Input: part model. Units: mm. Frame: model coordinates. Face numbers are marked on the shaded views. Give positions to 0.01 mm unless a question says otherwise; leave off trailing zeros. Write each loop counter-clockwise with the first axis right and the second up, starting at its lowest first coordinate (ties: lowest second). Pieces come first, ordered by that corner, then holes. Notation, with made-up numbers: (9.5, 75) - (22.5, 75) arc R36 ccw to (22.5, 109) - close; hole circle Ø4 at (14.25, -22). An arc over 180 degrees is marked (long way). Answer as CSV lines item,"result". Start each with the question number.
Autodesk Inventor part; units mm, degrees
ref_plane "YZ Plane" through (0, 0, 0) normal (1, 0, 0) x (0, 1, 0)
ref_plane "XZ Plane" through (0, 0, 0) normal (0, 1, 0) x (-1, 0, 0)
ref_plane "XY Plane" through (0, 0, 0) normal (0, 0, 1) x (1, 0, 0)
sketch "Sketch1" plane through (0, 0, 0) normal (0, 1, 0) x (-1, 0, 0)
  arc A0 (6.35, 25.4) -> (-6.35, 25.4) centre (0, 25.4) ccw
  arc A1 (-11.43, 15.24) -> (11.43, 15.24) centre (0, 0) ccw
  arc A2 (-11.43, 15.24) -> (-6.35, 25.4) centre (-19.05, 25.4) ccw
  arc A3 (6.35, 25.4) -> (11.43, 15.24) centre (19.05, 25.4) ccw
  dimension "d0" = 25.4
  dimension "d1" = 38.1
  dimension "d2" = 12.7
extrude "Extrusion1" add sketch "Sketch1" along normal blind 3.81
sketch "Sketch2" plane through (0, 3.81, 0) normal (0, 1, 0) x (1, 0, 0)
  arc A0 (-6.35, -25.4) -> (6.35, -25.4) centre (0, -25.4) ccw
  circle A1 centre (0, -25.4) radius 1.524
  dimension "d5" = 3.048
extrude "Extrusion2" cut sketch "Sketch2" against normal through all
pattern_circular "Circular Pattern1" count 3 over 360 about axis through (0, 0, 0) along (0, 1, 0) of "Extrusion2", "Extrusion1"
sketch "Sketch3" plane through (0, 3.81, 0) normal (0, 1, 0) x (1, 0, 0)
  arc A0 (11.43, -15.24) -> (18.9132, -2.2787) centre (0, 0) ccw
  line L0 (-10.2616, 10.6299) -> (7.3914, 10.6299)
  line L1 (7.3914, 10.6299) -> (7.3914, -11.7221)
  line L2 (7.3914, -11.7221) -> (-10.2616, -11.7221)
  line L3 (-10.2616, -11.7221) -> (-10.2616, 10.6299)
  dimension "d11" = 22.352
  dimension "d12" = 17.653
  dimension "d14" = 10.6299
  dimension "d29" = 7.3914
extrude "Extrusion3" cut sketch "Sketch3" against normal blind 2.54
sketch "Sketch4" plane through (0, 1.27, 0) normal (0, 1, 0) x (1, 0, 0)
  line L0 (-10.2616, 10.6299) -> (7.3914, 10.6299)
  line L1 (7.3914, -11.7221) -> (-10.2616, -11.7221)
  line L2 (7.3914, 10.6299) -> (7.3914, -11.7221)
  circle A0 centre (5.1816, 8.4201) radius 1.524
  circle A1 centre (5.1816, -9.5123) radius 1.524
  point P0 (0, 0)
  dimension "d17" = 3.048
  dimension "d18" = 2.2098
  dimension "d19" = 2.2098
  dimension "d20" = 2.2098
extrude "Extrusion4" cut sketch "Sketch4" against normal through all
sketch "Sketch5" plane through (0, 1.27, 0) normal (0, 1, 0) x (1, 0, 0)
  circle A0 centre (5.1816, 8.4201) radius 1.524
  circle A1 centre (5.1816, -9.5123) radius 1.524
  line L0 (-10.2616, 10.6299) -> (7.3914, 10.6299)
  circle A2 centre (5.1816, 8.4201) radius 3.175
  circle A3 centre (5.1816, -9.5123) radius 3.175
  point P0 (0, 0)
  dimension "d31" = 6.35
extrude "Extrusion5" add sketch "Sketch5" along normal blind 1.27
sketch "Sketch6" plane through (0, 3.81, 0) normal (0, 1, 0) x (1, 0, 0)
  line L0 (-10.2616, -11.7221) -> (-10.2616, 10.6299)
  line L1 (-10.2616, 10.6299) -> (7.3914, 10.6299)
  line L2 (-12.8016, 9.3599) -> (-12.8016, -3.3401)
  line L3 (-15.3416, -3.3401) -> (-15.3416, 9.3599)
  arc A0 (-12.8016, 9.3599) -> (-15.3416, 9.3599) centre (-14.0716, 9.3599) ccw
  arc A1 (-15.3416, -3.3401) -> (-12.8016, -3.3401) centre (-14.0716, -3.3401) ccw
  point P0 (-12.8016, -11.7221)
  dimension "d25" = 2.54
  dimension "d26" = 2.54
  dimension "d30" = 12.7
extrude "Extrusion6" cut sketch "Sketch6" against normal through all
equation "\"d19\" = d18"
equation "\"d20\" = d18"
properties part number "Gyro Mount"
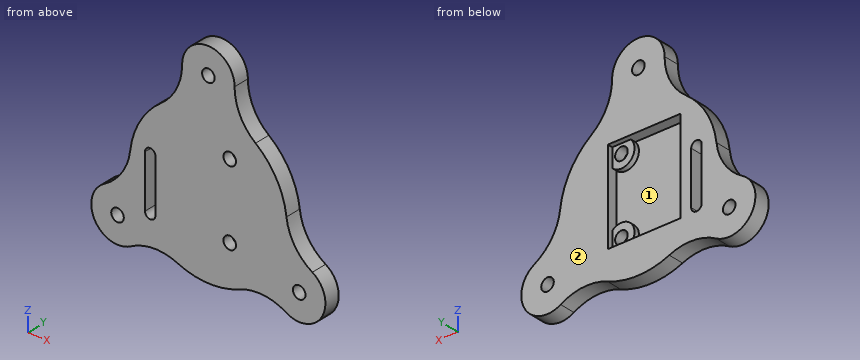
1) Material intervals for line 1 (X direction, y = 2.3, z = 10.5); line 2 (X direction, y = 1.6, z = 25.4); line 3 (Z direction, x = -14.5, y = 0.7), sorted ascending. Write a range as from..to.
2) Pull-direction query (X, two-part tool) for the marked faces 1 and 2; classes: +X half, -X half, draft (parallel to the pull), parting line (faces both ways), or undercut.
3) Contact query for flat-ended pins moving along their axis: P1, Ø1.3, axis at y = 3, z = 6, coming from the +X side; P2, Ø1.5, axis at y = 1.5, z = 16.5, coming from the -X side; P3, Ø4.5, axis at x = 4, z = -7, coming from the +Y side; P4, Ø5, axis at x = 5.18, z = 9.51, coming from the -Y side. Output: stop coordinate, or through.
4) Cut plane A-A on x = 0. Output: boundary loops of the cut face in (y, z), and give its area (3 significant figures).
5) Cut plane D-D on x = 13.5. Output: boundary loops of the cut face in (y, z).
6) Cut plane C-C on z = -0.5. Output: boundary loops of the cut face in (x, y).
7) Cut plane B-B on z = -12.7. Output: boundary loops of the cut face in (x, y), and give its area (3 significant figures).
Numbers:
1,line 1,"x = -15.9..-10.26, 2.16..4.02, 6.34..15.9"
1,line 2,"x = -6.35..-1.52, 1.52..6.35"
1,line 3,"z = -16.66..-10.56, 4.54..12.36"
2,face 1,"undercut"
2,face 2,"draft"
3,P1,"stops at x = 18.28"
3,P2,"stops at x = -10.79"
3,P3,"stops at y = 2.54"
3,P4,"stops at y = 0"
4,outline,"(0, -19.05) - (3.81, -19.05) - (3.81, -10.63) - (1.27, -10.63) - (1.27, 11.72) - (3.81, 11.72) - (3.81, 23.88) - (0, 23.88) - close; (0, 26.92) - (3.81, 26.92) - (3.81, 31.75) - (0, 31.75) - close"
4,area,"125 mm²"
5,outline,"(0, -16.54) - (3.81, -16.54) - (3.81, 13.44) - (0, 13.44) - close"
6,outline,"(-19.57, 0) - (-15.34, 0) - (-15.34, 3.81) - (-19.57, 3.81) - close; (-12.8, 0) - (19.57, 0) - (19.57, 3.81) - (7.39, 3.81) - (7.39, 1.27) - (-10.26, 1.27) - (-10.26, 3.81) - (-12.8, 3.81) - close"
7,outline,"(-28.35, 0) - (-23.52, 0) - (-23.52, 3.81) - (-28.35, 3.81) - close; (-20.47, 0) - (20.47, 0) - (20.47, 3.81) - (-20.47, 3.81) - close; (23.52, 0) - (28.35, 0) - (28.35, 3.81) - (23.52, 3.81) - close"
7,area,"193 mm²"
